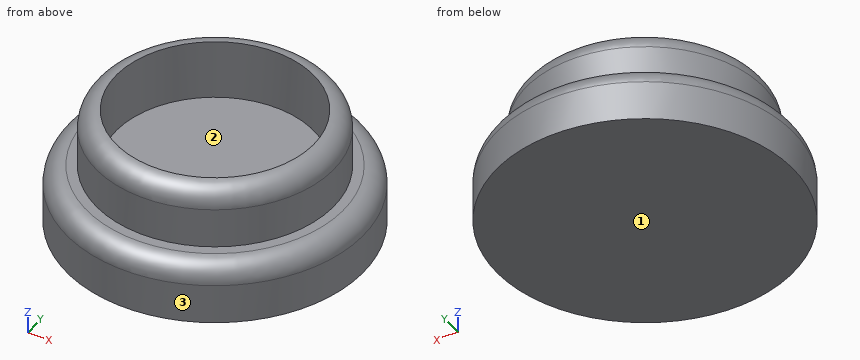
```python
from build123d import *

# Parameters (mm, degrees)
F0_R     = 7.5
F0_R_2   = 6
F0_R_3   = 5
F1_DEPTH = 3
F2_DEPTH = 3
F3_R     = 0.99999


# Not quite as in the source:
# - a fillet or chamfer is up to 0.001 mm smaller than in the source, because OpenCascade refuses the exact size


with BuildPart() as f1:
    # F0 (on Top) → F1 (new body)
    with BuildSketch(Plane.XY):
        Circle(F0_R)
        Circle(F0_R_2, mode=Mode.SUBTRACT)
        Circle(F0_R_2)
        Circle(F0_R_3, mode=Mode.SUBTRACT)
        Circle(F0_R_3)
    extrude(amount=-F1_DEPTH)

    # F0 (on Top) → F2 (join)
    with BuildSketch(Plane.XY):
        Circle(F0_R_2)
        Circle(F0_R_3, mode=Mode.SUBTRACT)
    extrude(amount=F2_DEPTH)

    # F3 (radius 1 in the source; OpenCascade refuses exactly that, so slightly less here)
    f3_edges = [f1.edges().sort_by_distance(p)[0] for p in [
        (-7.5, 0, 0),
        (-6, 0, 3),
    ]]
    fillet(f3_edges, radius=F3_R)


solid = f1.part
```
The listing builds one solid part. Answer for the finished solid, in the listing's coordinates (mm). Face numbers are marked on the shaded views. Round coordinates to 2 decimals unless told otherwise and drop trailing zeros. Write each loop counter-clockwise with the first axis right and the second up, starting at its lowest first coordinate (ties: lowest second). Pieces come first, ordered by that corner, then holes. Notation, with made-up numbers: (75.5, 73.25) -> (85.5, 73.25) arc R23 cw to (85.5, 103.25) -> close; hole circle Ø5 at (72, -13). An arc over 180 degrees is marked (long way). Answer as a JSON object with one key per item and string values. Group by question number.
Q1. This flat-tipped pin is pushed along its axis until it touches: pin 1 Ø3 at (x, y) = (2, -0.5) entering from +Z. Where does it stop, or does it pass through?
Q2. Section D-D (z = -1.7) is taken. Write down the section's boundary in (x, y).
Q3. Straight lines are drawn through the part: line 1 along Y through (x, z) = (0, 1.7); line 2 along Z through (x, y) = (-5.75, 2); line 3 along X through (y, z) = (0.25, 2.1). For each, find the intervals that lie inside material, in ascending order.
Q4. Determine the mould class of the marked faces 1, 2 and 3 for opening direction X: pulls with the +X half, pulls with the -X half, needs draft (parallel to the pull), parting line crosses it, or undercut.
Q5. Section C-C (z = 0.2) is taken. Write down the section's boundary in (x, y).
Check values:
{
 "1": {"pin 1": "z = 0"},
 "2": {"outline": "circle Ø15 at (0, 0)"},
 "3": {"line 1": "-6 to -5, 5 to 6", "line 2": "-3 to 0", "line 3": "-5.99 to -4.99, 4.99 to 5.99"},
 "4": {"face 1": "needs draft", "face 2": "undercut", "face 3": "parting line crosses it"},
 "5": {"outline": "circle Ø12 at (0, 0); hole circle Ø10 at (0, 0)"}
}
